```python
from build123d import *

# Parameters (mm, degrees)
SKETCH1_W           = 6.691688341
SKETCH1_H           = 7.98
SKETCH1_R           = 1.6
BOSS_EXTRUDE1_DEPTH = 5
SKETCH2_W           = 41.577195194
SKETCH2_H           = 43.078854614
BOSS_EXTRUDE2_DEPTH = 21.5
CUT_EXTRUDE1_DEPTH  = 6.691688
CUT_EXTRUDE2_START  = -65.83
CUT_EXTRUDE2_DEPTH  = 6.691688
RIB2_REACH          = 54.453
SKETCH4_WALL_W      = 115.956406408
SKETCH4_WALL_H      = 30


with BuildPart() as part:
    # Sketch1 → Boss-Extrude1 (new body)
    # profile 1 of 5: a face of its own
    with BuildSketch(Plane(origin=(0, 0, 0), x_dir=(1, 0, 0), z_dir=(0, 1, 0))):
        with Locations((-29.569155829, 21.5)):
            Rectangle(SKETCH1_W, SKETCH1_H)
        with Locations(Location((-29.915, 21.5, 0), (0, 0, 270))):
            Circle(SKETCH1_R, mode=Mode.SUBTRACT)
    # profile 2 of 5: a face of its own
    with BuildSketch(Plane(origin=(0, 0, 0), x_dir=(1, 0, 0), z_dir=(0, 1, 0))):
        with Locations((-29.569155829, -21.5)):
            Rectangle(SKETCH1_W, SKETCH1_H)
        with Locations(Location((-29.915, -21.5, 0), (0, 0, 270))):
            Circle(SKETCH1_R, mode=Mode.SUBTRACT)
    # profile 3 of 5: a face of its own
    with BuildSketch(Plane(origin=(0, 0, 0), x_dir=(1, 0, 0), z_dir=(0, 1, 0))):
        with BuildLine():
            Line((-26.223311659, 25.49), (-26.223311659, 17.51))
            Line((-26.223311659, 17.51), (-26.223311659, -17.51))
            Line((-26.223311659, -17.51), (-26.223311659, -25.49))
            ThreePointArc((-26.223311659, -25.49), (-24.173059128, -30.439747468), (-19.223311659, -32.49))
            Line((-19.223311659, -32.49), (19.223311659, -32.49))
            ThreePointArc((19.223311659, -32.49), (24.173059128, -30.439747468), (26.223311659, -25.49))
            Line((26.223311659, -25.49), (26.223311659, -17.51))
            Line((26.223311659, -17.51), (26.223311659, 17.51))
            Line((26.223311659, 17.51), (26.223311659, 25.49))
            ThreePointArc((26.223311659, 25.49), (24.173059128, 30.439747468), (19.223311659, 32.49))
            Line((19.223311659, 32.49), (-19.223311659, 32.49))
            ThreePointArc((-19.223311659, 32.49), (-24.173059128, 30.439747468), (-26.223311659, 25.49))
        make_face()
    # profile 4 of 5: a face of its own
    with BuildSketch(Plane(origin=(0, 0, 0), x_dir=(1, 0, 0), z_dir=(0, 1, 0))):
        with Locations((29.569155829, 21.5)):
            Rectangle(SKETCH1_W, SKETCH1_H)
        with Locations(Location((29.915, 21.5, 0), (0, 0, 270))):
            Circle(SKETCH1_R, mode=Mode.SUBTRACT)
    # profile 5 of 5: a face of its own
    with BuildSketch(Plane(origin=(0, 0, 0), x_dir=(1, 0, 0), z_dir=(0, 1, 0))):
        with Locations((29.569155829, -21.5)):
            Rectangle(SKETCH1_W, SKETCH1_H)
        with Locations(Location((29.915, -21.5, 0), (0, 0, 270))):
            Circle(SKETCH1_R, mode=Mode.SUBTRACT)
    extrude(amount=BOSS_EXTRUDE1_DEPTH)

    # Sketch2 → Boss-Extrude2 (add)
    with BuildSketch(Plane.XZ):
        with Locations((-2.205562273, 0)):
            Rectangle(SKETCH2_W, SKETCH2_H)
    extrude(amount=BOSS_EXTRUDE2_DEPTH)

    # Sketch3 → Cut-Extrude1 (cut)
    with BuildSketch(Plane.ZY.offset(32.915)):
        Polygon((-18.304058028, 3.156143774), (-17.51, 3.156143774), (-17.51, 5), (-25.49, 5), (-25.49, 3.156143774), (-24.695941972, 3.156143774), (-24.695941972, 1.28299036), (-18.304058028, 1.28299036), align=None)
        Polygon((24.695941972, 3.156143774), (25.49, 3.156143774), (25.49, 5), (17.51, 5), (17.51, 3.156143774), (18.304058028, 3.156143774), (18.304058028, 1.28299036), (24.695941972, 1.28299036), align=None)
    extrude(amount=-CUT_EXTRUDE1_DEPTH, mode=Mode.SUBTRACT)

    # Sketch3<3> → Cut-Extrude2 (cut)
    with BuildSketch(Plane.ZY.offset(32.915).offset(CUT_EXTRUDE2_START)):
        Polygon((24.695941972, 3.156143774), (25.49, 3.156143774), (25.49, 5), (17.51, 5), (17.51, 3.156143774), (18.304058028, 3.156143774), (18.304058028, 1.28299036), (24.695941972, 1.28299036), align=None)
        Polygon((-18.304058028, 3.156143774), (-17.51, 3.156143774), (-17.51, 5), (-25.49, 5), (-25.49, 3.156143774), (-24.695941972, 3.156143774), (-24.695941972, 1.28299036), (-18.304058028, 1.28299036), align=None)
    extrude(amount=CUT_EXTRUDE2_DEPTH, mode=Mode.SUBTRACT)

    # Sketch4 wall → Rib2 (add, up to next)
    with BuildSketch(Plane(origin=(-2.205562273, -2.161622642, -25.515102301), x_dir=(0, 0.477671912918, -0.878538299455), z_dir=(0, 0.878538299455, 0.477671912918)), mode=Mode.PRIVATE) as rib2_sk1:
        Rectangle(SKETCH4_WALL_W, SKETCH4_WALL_H)
    rib2_tool1 = extrude(rib2_sk1.sketch, amount=RIB2_REACH, mode=Mode.PRIVATE) - part.part
    rib2 = rib2_tool1.solids().sort_by_distance((-2.205562273, -2.161622642, -25.515102301))[0]
    add(rib2)

    # Mirror4: Rib2 across plane
    add(rib2.mirror(Plane.XY))


solid = part.part
```
Geometry: final body of the model. Coordinates: model frame, mm. A direction names the side the tool comes from. Coordinates: 2 decimals unless noted, no trailing zeros. Loops run counter-clockwise (first coordinate to the right, second up) from the corner with the lowest first, then second, coordinate; pieces in that order, holes last. Notation, with made-up numbers: (85, 34) -> (101, 34) arc R20 cw to (101, 55) -> close; hole circle Ø10 at (72.5, 44.5). An arc over 180 degrees is marked (long way). Use a Markdown table: item, result. Add a question column.
(1) Line query: line 1 along X through (y, z) = (0.5, -21.5) (3 decimals); line 2 along Y through (x, z) = (22, 20.5); line 3 along Z through (x, y) = (3, -4.75). Output: solid intervals per line, ascending.
(2) Access query for faces 1 (the flat face through (-30, 2, -18.304)), 2 (the flat face through (-2, -21.5, 0)), 3 (the flat face through (-22.994, -11, 0)), 4 (the flat face through (-17.206, -2, 24)), 5 (the flat face through (28, 1.283, 21)). Directions: +Z, -Z, +X, -X, +Y, -Y. A direction counts if a zero-diameter tool reaches every point of the face in a straight line with its end or side. Return the directions, or none.
(3) Section query C-C, the plane x = 20.5. Return loops of the section in (y, z), plus the area to 3 significant figures.
(4) Mould query, pull axis Z, two halves, no side actions, for faces 6 (the cylindrical face through (24.227, 2.465, -30.385)), 7 (the flat face through (-30, 1, 25.49)), 8 (the flat face through (19, 0, 0)), 9 (the flat face through (-26.223, 3, 21)). Classes: pulls with the +Z half, pulls with the -Z half, needs draft (parallel to the pull), parting line crosses it, or undercut.
(5) Section query A-A, the plane z = 10. Return loops of the section in (x, y), plus the area to 3 significant figures.
(6) Pin query (flat end, axial travel): pin 1 Ø2 at (y, z) = (-1.5, -13) entering from -X; pin 2 Ø2.5 at (x, y) = (30, 2) entering from -Z; pin 3 Ø5 at (x, z) = (-30.5, -21.5) entering from +Y. Return the tip coordinate at first contact, or that it passes through.
(7) Section query B-B, the plane x = 10. Return loops of the section in (y, z), plus the area to 3 significant figures.
Answer:
| question | item | result |
|---|---|---|
| 1 | line 1 | x = -32.915 to -31.515, -28.315 to 28.315, 31.515 to 32.915 |
| 1 | line 2 | y = 0 to 5 |
| 1 | line 3 | z = -21.54 to 21.54 |
| 2 | face 1 | -X, +Y |
| 2 | face 2 | +Z, -Z, +X, -X, -Y |
| 2 | face 3 | +Z, -Z, -X, -Y |
| 2 | face 4 | +Z, -X, -Y |
| 2 | face 5 | +X, +Y |
| 3 | outline | (0, -32.37) -> (5, -32.37) -> (5, 32.37) -> (0, 32.37) -> close |
| 3 | area | 324 mm^2 |
| 4 | face 6 | pulls with the -Z half |
| 4 | face 7 | pulls with the +Z half |
| 4 | face 8 | needs draft |
| 4 | face 9 | undercut |
| 5 | outline | (-26.22, 0) -> (-22.99, 0) -> (-22.99, -21.5) -> (18.58, -21.5) -> (18.58, 0) -> (26.22, 0) -> (26.22, 5) -> (-26.22, 5) -> close |
| 5 | area | 1,160 mm^2 |
| 6 | pin 1 | stops at x = -22.99 |
| 6 | pin 2 | stops at z = -25.49 |
| 6 | pin 3 | stops at y = 1.28 |
| 7 | outline | (-21.5, -21.54) -> (-4.32, -21.54) -> (0, -29.49) -> (0, -32.49) -> (5, -32.49) -> (5, 32.49) -> (0, 32.49) -> (0, 29.49) -> (-4.32, 21.54) -> (-21.5, 21.54) -> close |
| 7 | area | 1,290 mm^2 |
